Source: CAD feature listing. Evaluate the final solid. Frame: model axes, mm. Face numbers are marked on the shaded views. A direction names the side the tool comes from. Give positions to 0.01 mm unless a question says otherwise; leave off trailing zeros. Write each loop counter-clockwise with the first axis right and the second up, starting at its lowest first coordinate (ties: lowest second). Pieces come first, ordered by that corner, then holes. Notation, with made-up numbers: (20.25, 72.5) -> (41.25, 72.5) arc R20 ccw to (41.25, 101.5) -> close; hole circle Ø2 at (-34, -17.5). An arc over 180 degrees is marked (long way). Write item = value, one per line.
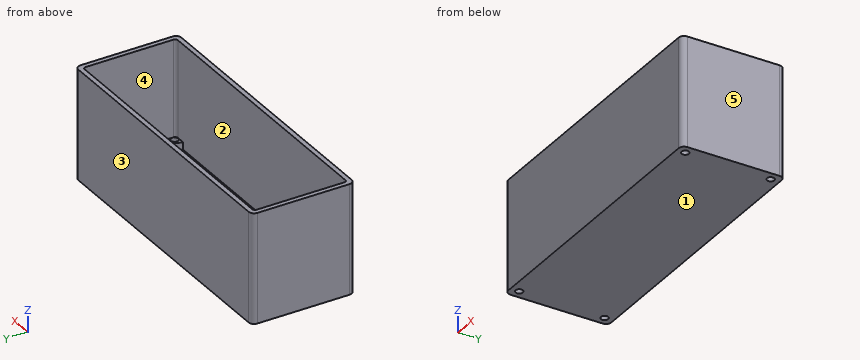
from build123d import *

# Parameters (mm, degrees)
F1_DEPTH = 40.64
F3_DEPTH = 38.608
F5_DEPTH = 4.7752
F6_R     = 1.35255
F7_DEPTH = 4.7752


# Not quite as in the source:
# - a feature names something its author has since deleted; it is built from what else it names


with BuildPart() as f1:
    # F0 (on Top) → F1 (new body)
    with BuildSketch(Plane.XY):
        with BuildLine():
            ThreePointArc((0, 2), (0.5857864376, 0.5857864376), (2, 0))
            Line((2, 0), (105.061, 0))
            ThreePointArc((105.061, 0), (106.4752135624, 0.5857864376), (107.061, 2))
            Line((107.061, 2), (107.061, 36.1))
            ThreePointArc((107.061, 36.1), (106.4752135624, 37.5142135624), (105.061, 38.1))
            Line((105.061, 38.1), (2, 38.1))
            ThreePointArc((2, 38.1), (0.5857864376, 37.5142135624), (0, 36.1))
            Line((0, 36.1), (0, 2))
        make_face()
    extrude(amount=F1_DEPTH)

    # F2 (on face) → F3 (cut)
    with BuildSketch(Plane.XY.offset(40.64)):
        with BuildLine():
            Line((104.261, 36.3), (2.8, 36.3))
            ThreePointArc((2.8, 36.3), (2.0928932188, 36.0071067812), (1.8, 35.3))
            Line((1.8, 35.3), (1.8, 2.8))
            ThreePointArc((1.8, 2.8), (2.0928932188, 2.0928932188), (2.8, 1.8))
            Line((2.8, 1.8), (104.261, 1.8))
            ThreePointArc((104.261, 1.8), (104.9681067812, 2.0928932188), (105.261, 2.8))
            Line((105.261, 2.8), (105.261, 35.3))
            ThreePointArc((105.261, 35.3), (104.9681067812, 36.0071067812), (104.261, 36.3))
        make_face()
    extrude(amount=-F3_DEPTH, mode=Mode.SUBTRACT)

    # F4 (on face) → F5 (join)
    with BuildSketch(Plane(origin=(0, 0, 0), x_dir=(1, 0, 0), z_dir=(0, 0, -1))):
        with BuildLine():
            ThreePointArc((107.061, -2), (106.4752135624, -0.5857864376), (105.061, 0))
            Line((105.061, 0), (101.251, 0))
            Line((101.251, 0), (101.251, -2))
            ThreePointArc((101.251, -2), (102.3669231637, -4.6940768363), (105.061, -5.81))
            Line((105.061, -5.81), (107.061, -5.81))
            Line((107.061, -5.81), (107.061, -2))
        make_face()
        with BuildLine():
            Line((101.251, -36.1), (101.251, -38.1))
            Line((101.251, -38.1), (105.061, -38.1))
            ThreePointArc((105.061, -38.1), (106.4752135624, -37.5142135624), (107.061, -36.1))
            Line((107.061, -36.1), (107.061, -32.29))
            Line((107.061, -32.29), (105.061, -32.29))
            ThreePointArc((105.061, -32.29), (102.3669231637, -33.4059231637), (101.251, -36.1))
        make_face()
        with BuildLine():
            ThreePointArc((5.81, -36.1), (4.6940768363, -33.4059231637), (2, -32.29))
            Line((2, -32.29), (0, -32.29))
            Line((0, -32.29), (0, -36.1))
            ThreePointArc((0, -36.1), (0.5857864376, -37.5142135624), (2, -38.1))
            Line((2, -38.1), (5.81, -38.1))
            Line((5.81, -38.1), (5.81, -36.1))
        make_face()
        with BuildLine():
            Line((5.81, 0), (2, 0))
            ThreePointArc((2, 0), (0.5857864376, -0.5857864376), (0, -2))
            Line((0, -2), (0, -5.81))
            Line((0, -5.81), (2, -5.81))
            ThreePointArc((2, -5.81), (4.6940768363, -4.6940768363), (5.81, -2))
            Line((5.81, -2), (5.81, 0))
        make_face()
    extrude(amount=-F5_DEPTH)

    # F6 (on face) → F7 (cut, through all)
    with BuildSketch(Plane(origin=(0, 0, 0), x_dir=(1, 0, 0), z_dir=(0, 0, -1))):
        with Locations((103.8037641431, -3.2572358569)):
            Circle(F6_R)
        with Locations((3.2572358569, -3.2572358569)):
            Circle(F6_R)
        with Locations((3.2572358569, -34.8427641431)):
            Circle(F6_R)
        with Locations((103.8037641431, -34.8427641431)):
            Circle(F6_R)
    extrude(amount=-F7_DEPTH, mode=Mode.SUBTRACT)


solid = f1.part
(1) Section query C-C (y = 26.5). Return loops of the section in (x, z).
Values follow:
outline = (0, 0) -> (107.06, 0) -> (107.06, 40.64) -> (105.26, 40.64) -> (105.26, 2.03) -> (1.8, 2.03) -> (1.8, 40.64) -> (0, 40.64) -> close
(2) Pull-direction query (X, two-part tool) for the marked faces 3, 4 and 5; classes: pulls with the +X half, pulls with the -X half, needs draft (parallel to the pull), parting line crosses it, or undercut.
Values follow:
face_3 = needs draft
face_4 = undercut
face_5 = pulls with the +X half
(3) Access query for the marked faces 1 and 2. Directions: +Z, -Z, +X, -X, +Y, -Y. A direction counts if a zero-diameter tool reaches every point of the face in a straight line with its end or side. Return the directions, or none.
Values follow:
face_1 = -Z, +X, -X, +Y, -Y
face_2 = +Z
(4) Section query A-A (z = 24). Return loops of the section in (x, y), plus the area to 3 significant figures.
Values follow:
outline = (0, 2) arc R2 ccw to (2, 0) -> (105.06, 0) arc R2 ccw to (107.06, 2) -> (107.06, 36.1) arc R2 ccw to (105.06, 38.1) -> (2, 38.1) arc R2 ccw to (0, 36.1) -> close; hole (1.8, 2.8) arc R1 ccw to (2.8, 1.8) -> (104.26, 1.8) arc R1 ccw to (105.26, 2.8) -> (105.26, 35.3) arc R1 ccw to (104.26, 36.3) -> (2.8, 36.3) arc R1 ccw to (1.8, 35.3) -> close
area = 507 mm2
(5) Material intervals for line 1 (Y direction, x = 67, z = 9.5); line 2 (X direction, y = 9, z = 29); line 3 (X direction, y = 35.5, z = 21.5), sorted ascending.
Values follow:
line_1 = 0 to 1.8, 36.3 to 38.1
line_2 = 0 to 1.8, 105.26 to 107.06
line_3 = 0 to 1.82, 105.24 to 107.06
(6) Section query B-B (x = 26). Return loops of the section in (y, z).
Values follow:
outline = (0, 0) -> (38.1, 0) -> (38.1, 40.64) -> (36.3, 40.64) -> (36.3, 2.03) -> (1.8, 2.03) -> (1.8, 40.64) -> (0, 40.64) -> close
(7) First-contact query: pin 1 (6 mm diameter, centred on x = 67, y = 30, fed in from +Z); pin 2 (1.2 mm diameter, centred on x = 3, y = 4.5, fed in from +Z). Flat tips, straight axial feed; report the tip coordinate or a pass-through.
Values follow:
pin_1 = 2.03
pin_2 = 4.78
